Drawing for the job (mm, zero at the part's lowest x, y, z). A direction names the side the tool comes from. Round coordinates to 2 decimals unless told otherwise and drop trailing zeros. Loops run counter-clockwise (first coordinate to the right, second up) from the corner with the lowest first, then second, coordinate; pieces in that order, holes last. Notation, with made-up numbers: (-18, -32.5) -> (-1, -32.5) arc R27 ccw to (-1, 5.5) -> close; hole circle Ø7 at (82.5, 19.5). An arc over 180 degrees is marked (long way). Put each result on its own line as item: value. Start each with the question number.
Item 1: Tool access for the marked faces 1 and 2: list every direction of +Z, -Z, +X, -X, +Y, -Y with a clear straight run to the whole face (end or side of a thin tool).
Item 2: Pull direction X, two halves, no side cores. Call the marked faces 3, 4 and 5: +X half, -X half, draft (parallel to the pull), parting line (faces both ways), or undercut.
Item 3: Cut at A-A, the plane z = 33.5. List the corners of the cut face in (x, y), plus the area to 3 significant figures.
Item 4: Cut at D-D, the plane y = 35. List the corners of the cut face in (x, z).
Item 5: Drill centre lines: probe 1 along Z at (x, y) = (112, 10) (1 decimal); probe 2 along X at (y, z) = (3, 49.5); probe 3 along Y at (x, z) = (2.3, 7.1). Where is each one in solid material? Low to high. Write a range as [from, to].
Item 6: Cut at C-C, the plane y = 48.5. List the corners of the cut face in (x, z).
Item 7: Flat gauge pins, fed straight in: pin 1 Ø16.5 at (x, z) = (86, 35) entering from -Y; pin 2 Ø5 at (x, y) = (99, 29) entering from -Z. Where does each tip first touch, or does it go through?
Item 8: Cut at B-B, the plane x = 89. List the corners of the cut face in (y, z).
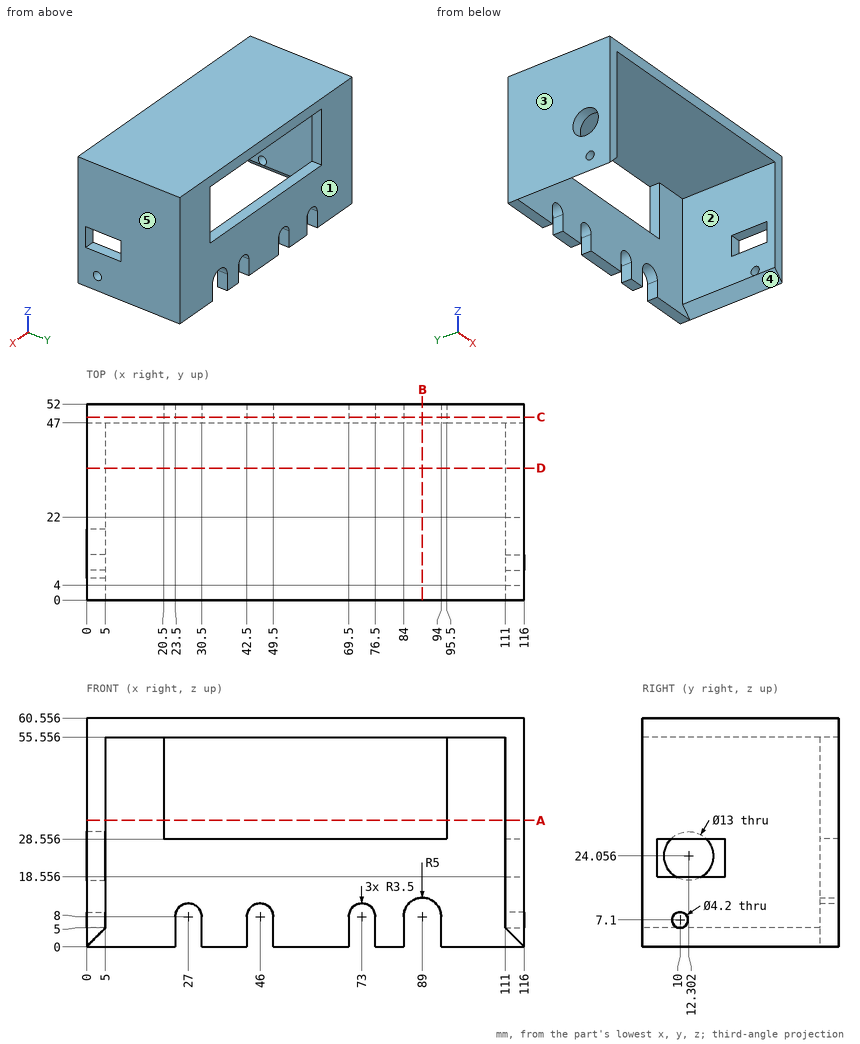
Reply:
1. face 1: +Z, -Z, +X, -X, +Y
1. face 2: -Z, -Y
2. face 3: -X half
2. face 4: undercut
2. face 5: +X half
3. outline: (0, 0) -> (5, 0) -> (5, 47) -> (20.5, 47) -> (20.5, 52) -> (0, 52) -> close; (95.5, 47) -> (111, 47) -> (111, 0) -> (116, 0) -> (116, 52) -> (95.5, 52) -> close
3. area: 675 mm^2
4. outline: (0, 0) -> (5, 5) -> (5, 55.56) -> (111, 55.56) -> (111, 5) -> (116, 0) -> (116, 60.56) -> (0, 60.56) -> close
5. probe 1: z = [4, 5], [9.2, 18.6], [28.6, 60.6]
5. probe 2: x = [0, 5], [111, 116]
5. probe 3: y = [0, 7.9], [12.1, 52]
6. outline: (0, 0) -> (23.5, 0) -> (23.5, 8) arc R3.5 cw to (30.5, 8) -> (30.5, 0) -> (42.5, 0) -> (42.5, 8) arc R3.5 cw to (49.5, 8) -> (49.5, 0) -> (69.5, 0) -> (69.5, 8) arc R3.5 cw to (76.5, 8) -> (76.5, 0) -> (84, 0) -> (84, 8) arc R5 cw to (94, 8) -> (94, 0) -> (116, 0) -> (116, 60.56) -> (0, 60.56) -> close; hole (20.5, 28.56) -> (95.5, 28.56) -> (95.5, 55.56) -> (20.5, 55.56) -> close
7. pin 1: stops at y = 47
7. pin 2: stops at z = 55.56
8. outline: (0, 55.56) -> (52, 55.56) -> (52, 60.56) -> (0, 60.56) -> close; (47, 13) -> (52, 13) -> (52, 28.56) -> (47, 28.56) -> close
